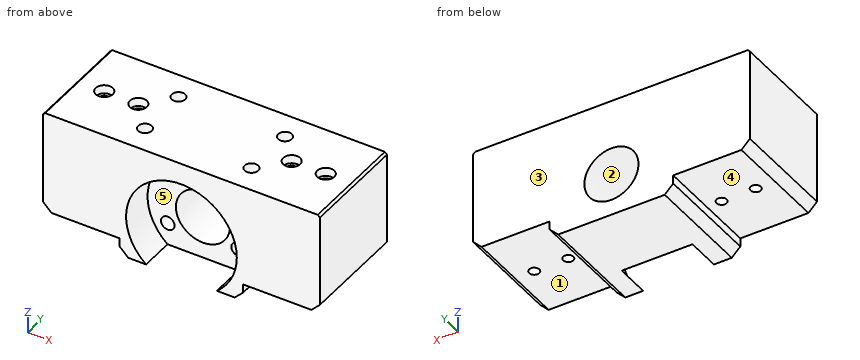
```python
from build123d import *

# Parameters (mm, degrees)
F0_R           = 6.35
F1_DEPTH       = 25
F2_SIZE        = 0.5
F3_R           = 6.35
F4_DEPTH       = 8
F5_SIZE        = 2
F7_D           = 3.2
F7_DEPTH       = 8
F7_TIP         = 0.9613769904
F9_D           = 2.4
F9_CBORE_D     = 4
F9_CBORE_DEPTH = 2
F11_D          = 3.2
F11_DEPTH      = 10
F11_TIP        = 0.9613769904


with BuildPart() as f1:
    # F0 (on Front) → F1 (new body)
    with BuildSketch(Plane.XZ):
        Polygon((-14.5, -10), (14.5, -10), (14.5, -6), (32.5, -6), (32.5, 18), (-32.5, 18), (-32.5, -6), (-14.5, -6), align=None)
        Circle(F0_R, mode=Mode.SUBTRACT)
    extrude(amount=F1_DEPTH)

    # F2
    f2_edges = [f1.edges().sort_by_distance(p)[0] for p in [
        (-32.5, -12.5, 18),
        (32.5, -12.5, 18),
    ]]
    chamfer(f2_edges, length=F2_SIZE)

    # F3 (on face) → F4 (cut)
    with BuildSketch(Plane.XZ.offset(25)):
        with BuildLine():
            ThreePointArc((8.3066238629, -10), (11.7683072321, -5.5233092337), (13, 0))
            ThreePointArc((13, 0), (-5.5233092337, 11.7683072321), (-8.3066238629, -10))
            Line((-8.3066238629, -10), (8.3066238629, -10))
        make_face()
        Circle(F3_R, mode=Mode.SUBTRACT)
    extrude(amount=-F4_DEPTH, mode=Mode.SUBTRACT)

    # F5
    f5_edges = [f1.edges().sort_by_distance(p)[0] for p in [
        (32.5, -12.5, -6),
        (14.5, -12.5, -10),
        (-14.5, -12.5, -10),
        (-32.5, -12.5, -6),
    ]]
    chamfer(f5_edges, length=F5_SIZE)

    # F7
    with Locations(Plane.XY.offset(18)):
        with Locations((12.5, -6.25), (12.5, -18.75), (-12.5, -6.25), (-12.5, -18.75)):
            Hole(F7_D / 2, depth=F7_DEPTH)
            with Locations((0, 0, -(F7_DEPTH + F7_TIP / 2))):  # 118° drill point
                Cone(0, F7_D / 2, F7_TIP, mode=Mode.SUBTRACT)

    # F9 (through all)
    with Locations(Plane.XY.offset(18)):
        with Locations((-26, -12.5), (-18, -12.5), (18, -12.5), (26, -12.5)):
            CounterBoreHole(F9_D / 2, F9_CBORE_D / 2, F9_CBORE_DEPTH)

    # F11
    with Locations(Plane.XZ.offset(17)):
        with Locations((0, 9.53), (8.2532220981, -4.765), (-8.2532220981, -4.765)):
            Hole(F11_D / 2, depth=F11_DEPTH)
            with Locations((0, 0, -(F11_DEPTH + F11_TIP / 2))):  # 118° drill point
                Cone(0, F11_D / 2, F11_TIP, mode=Mode.SUBTRACT)


solid = f1.part
```
Read the model definition and answer for the solid it produces. Units are mm, in the model's axes. Face numbers are marked on the shaded views. A direction names the side the tool comes from. Give positions to 0.01 mm unless a question says otherwise; leave off trailing zeros. Order: outer loops, then holes, each group sorted by start corner. A loop starts at its lowest first (then second) coordinate and runs counter-clockwise, first axis right, second up.
(1) Given pin 1 (4 mm diameter, centred on x = -18, y = -12.5, fed in from -Z); pin 2 (1.2 mm diameter, centred on x = -17.5, y = -13.5, fed in from +Z); pin 3 (1 mm diameter, centred on y = -7.5, z = -7, fed in from +X), each flat-ended and moving along its own axis, determine where each tip first touches the part or whether it passes through.
(2) Find section A-A (x = -26). Give the vertices of the cut face in (y, z), plus the area to 3 significant figures.
(3) Straight lines are drawn through the part: L1, parallel to Y at x = -12.5, z = 13.75; L2, parallel to Z at x = 0, y = -11.5; L3, parallel to X at y = -6.25, z = 16.25. For each, find the intervals that lie inside material, in ascending order.
(4) Find section C-C (y = -12.5). Give the number of separate pieces and of enclosed holes in the cut face, plus the area to 3 significant figures.
(5) Find section B-B (z = 1). Give the vertices of the cut face in (x, y).
(6) For the marked faces 1, 2, 3, 4 and 5, determine the directions among +Z, -Z, +X, -X, +Y, -Y from which every point of the face is accessible in a straight line to the end or side of a thin tool.
(7) Find section D-D (x = 21.5). Give the vertices of the cut face in (y, z).
Result sheet:
1. pin 1: stops at z = -6
1. pin 2: stops at z = 16
1. pin 3: stops at x = 14.5
2. outline: (-25, -6) - (-13.7, -6) - (-13.7, 16) - (-14.5, 16) - (-14.5, 18) - (-25, 18) - close; (-11.3, -6) - (0, -6) - (0, 18) - (-10.5, 18) - (-10.5, 16) - (-11.3, 16) - close
2. area: 539 mm2
3. L1: y = -25 to -20.35, -17.15 to -7.85, -4.65 to 0
3. L2: z = -10 to -6.35, 6.35 to 7.93, 11.13 to 18
3. L3: x = -32.5 to -14.1, -10.9 to 10.9, 14.1 to 32.5
4. separate pieces: 5
4. enclosed holes: 4
4. area: 1,270 mm2
5. outline: (-32.5, -25) - (-12.96, -25) - (-12.96, -17) - (-6.27, -17) - (-6.27, 0) - (-32.5, 0) - close; (6.27, -17) - (12.96, -17) - (12.96, -25) - (32.5, -25) - (32.5, 0) - (6.27, 0) - close; hole circle Ø2.4 at (-26, -12.5); hole circle Ø2.4 at (-18, -12.5); hole circle Ø2.4 at (18, -12.5); hole circle Ø2.4 at (26, -12.5)
6. face 1: -Z, +X, +Y, -Y
6. face 2: +Y, -Y
6. face 3: +Z, -Z, +X, -X, +Y
6. face 4: -Z, -X, +Y, -Y
6. face 5: -Y
7. outline: (-25, -6) - (0, -6) - (0, 18) - (-25, 18) - close
